Read the model definition and answer for the solid it produces. Units are mm, in the model's axes. A direction names the side the tool comes from. Give positions to 0.01 mm unless a question says otherwise; leave off trailing zeros. Loops run counter-clockwise (first coordinate to the right, second up) from the corner with the lowest first, then second, coordinate; pieces in that order, holes last. Notation, with made-up numbers: (-20.5, 8) - (26.5, 8) arc R17 cw to (26.5, 14) - close; hole circle Ø5 at (34, 47.5). An arc over 180 degrees is marked (long way). Write each question's results on one line, items separated by ' | '. Start each with the question number.
Q1. The part is cut by section A-A, the plane z = 121. Write down the section's boundary in (x, y) (3 decimals), plus the area to 3 significant figures.
Q2. Determine the mould class of faces 3 (the flat face through (1, 6, -127.5)), 4 (the flat face through (-67.875, 6, -2)), 5 (the flat face through (7, 9, -35.25)) for opening direction Z: +Z half, -Z half, draft (parallel to the pull), parting line (faces both ways), or undercut.
Q3. Given pin 1 (3 mm diameter, centred on x = -61, z = -121.5, fed in from +Y); pin 2 (3 mm diameter, centred on x = 33.5, z = -30, fed in from +Y); pin 3 (8 mm diameter, centred on x = -45, z = 54.175, fed in from +Y); pin 4 (5 mm diameter, centred on x = 45.5, z = 55, fed in from +Y), each flat-ended and moving along its own axis, determine where each tip first touches the part or whether it passes through.
Q4. Find the intervals of material crossed by line 1 (X direction, y = 4.55, z = 30) (3 decimals); line 2 (X direction, y = 7.5, z = 121) (3 decimals); line 3 (Z direction, x = 19, y = 5.25), in increasing order. Write a range as from..to.
Q5. For faces 1 (the flat face through (-45, 5.5, -54)), 2 (the flat face through (-31, 11.5, -2)), determine the directions among +Z, -Z, +X, -X, +Y, -Y from which every point of the face is accessible in a straight line to the end or side of a thin tool.
Q6. The part is cut by section C-C, the plane x = 1.5. Write down the section's boundary in (y, z).
Q7. The part is cut by section B-B, the plane x = -45. Write down the section's boundary in (y, z).
```python
from build123d import *

# Parameters (mm, degrees)
BOSS_EXTRUDE1_DEPTH     = 11.5
SKETCH4_R               = 3.075
CUT_EXTRUDE1_DEPTH      = 6
CUT_EXTRUDE6_DEPTH      = 4.6
CUT_EXTRUDE3_DEPTH      = 145.605932192
CUT_EXTRUDE3_DEPTH_BACK = 3.7
SKETCH24_W              = 82.375
SKETCH24_H              = 54
SKETCH25_R              = 1.35
CUT_EXTRUDE4_DEPTH      = 5
CHAMFER4_SIZE           = 0.5
FILLET1_R               = 2
BOSS_EXTRUDE2_DEPTH     = 0.8
CHAMFER5_SIZE           = 0.75


with BuildPart() as part:
    # Sketch1 → Boss-Extrude1 (new body)
    with BuildSketch(Plane(origin=(0, 0, 0), x_dir=(1, 0, 0), z_dir=(0, 1, 0))):
        with BuildLine():
            Line((-67.875, 112.5), (-67.875, -112.5))
            Line((-67.875, -112.5), (-67.875, -125.5))
            ThreePointArc((-67.875, -125.5), (-67.289213562, -126.914213562), (-65.875, -127.5))
            Line((-65.875, -127.5), (65.875, -127.5))
            ThreePointArc((65.875, -127.5), (67.289213562, -126.914213562), (67.875, -125.5))
            Line((67.875, -125.5), (67.875, -112.5))
            Line((67.875, -112.5), (67.875, 112.5))
            Line((67.875, 112.5), (67.875, 125.5))
            ThreePointArc((67.875, 125.5), (67.289213562, 126.914213562), (65.875, 127.5))
            Line((65.875, 127.5), (-65.875, 127.5))
            ThreePointArc((-65.875, 127.5), (-67.289213562, 126.914213562), (-67.875, 125.5))
            Line((-67.875, 125.5), (-67.875, 112.5))
        make_face()
    extrude(amount=BOSS_EXTRUDE1_DEPTH)

    # Sketch4 → Cut-Extrude1 (cut)
    with BuildSketch(Plane(origin=(0, 11.5, 0), x_dir=(1, 0, 0), z_dir=(0, 1, 0))):
        with Locations(Location((-59.875, -121, 0), (0, 0, 270))):
            Circle(SKETCH4_R)
        with Locations(Location((59.875, -121, 0), (0, 0, 270))):
            Circle(SKETCH4_R)
        with Locations(Location((59.875, 121, 0), (0, 0, 270))):
            Circle(SKETCH4_R)
        with Locations(Location((-59.875, 121, 0), (0, 0, 270))):
            Circle(SKETCH4_R)
        with Locations(Location((45, -54.175, 0), (0, 0, 270))):
            Circle(SKETCH4_R)
        with Locations(Location((-45, -54.175, 0), (0, 0, 270))):
            Circle(SKETCH4_R)
        with Locations(Location((45, 54.175, 0), (0, 0, 270))):
            Circle(SKETCH4_R)
        with Locations(Location((-45, 54.175, 0), (0, 0, 270))):
            Circle(SKETCH4_R)
    extrude(amount=-CUT_EXTRUDE1_DEPTH, mode=Mode.SUBTRACT)

    # Sketch21 → Cut-Extrude6 (cut)
    with BuildSketch(Plane(origin=(0, 11.5, 0), x_dir=(1, 0, 0), z_dir=(0, 1, 0))):
        Polygon((67.875, 31), (67.875, -31), (67.875, -31.25), (42.603553391, -31.25), (38.603553391, -35.25), (-22.75, -35.25), (-22.75, 35.25), (38.603553391, 35.25), (42.603553391, 31.25), (67.875, 31.25), align=None)
    extrude(amount=-CUT_EXTRUDE6_DEPTH, mode=Mode.SUBTRACT)

    # Sketch24 → Cut-Extrude3 (cut, two sides: drawn at the far end of the back side and taken through both)
    with BuildSketch(Plane(origin=(0, 6.9, 0), x_dir=(1, 0, 0), z_dir=(0, 1, 0)).offset(-CUT_EXTRUDE3_DEPTH_BACK)):
        with Locations((26.6875, 0)):
            Rectangle(SKETCH24_W, SKETCH24_H)
    extrude(amount=CUT_EXTRUDE3_DEPTH + CUT_EXTRUDE3_DEPTH_BACK, mode=Mode.SUBTRACT)

    # Sketch25 → Cut-Extrude4 (cut)
    with BuildSketch(Plane(origin=(0, 6.9, 0), x_dir=(1, 0, 0), z_dir=(0, 1, 0))):
        with Locations(Location((33.5, 30, 0), (0, 0, 270))):
            Circle(SKETCH25_R)
        with Locations(Location((-17.5, 30, 0), (0, 0, 270))):
            Circle(SKETCH25_R)
        with Locations(Location((33.5, -30, 0), (0, 0, 270))):
            Circle(SKETCH25_R)
        with Locations(Location((-17.5, -30, 0), (0, 0, 270))):
            Circle(SKETCH25_R)
    extrude(amount=-CUT_EXTRUDE4_DEPTH, mode=Mode.SUBTRACT)

    # Chamfer4
    chamfer4_edges = [part.edges().sort_by_distance(p)[0] for p in [
        (-17.5, 6.9, -31.35),
        (33.5, 6.9, 28.65),
        (-17.5, 6.9, 28.65),
        (33.5, 6.9, -31.35),
    ]]
    chamfer(chamfer4_edges, length=CHAMFER4_SIZE)

    # Fillet1
    fillet1_edges = [part.edges().sort_by_distance(p)[0] for p in [
        (26.6875, 3.2, -27),
        (-14.5, 5.05, -27),
        (-14.5, 3.2, 0),
        (-14.5, 5.05, 27),
        (26.6875, 3.2, 27),
    ]]
    fillet(fillet1_edges, radius=FILLET1_R)

    # Sketch26 → Boss-Extrude2 (add)
    with BuildSketch(Plane(origin=(0, 6.9, 0), x_dir=(1, 0, 0), z_dir=(0, 1, 0))):
        Polygon((38.603553391, 35.25), (38.603553391, 27), (67.875, 27), (67.875, 31.25), (42.603553391, 31.25), align=None)
        Polygon((42.603553391, -31.25), (38.603553391, -35.25), (38.603553391, -27), (67.875, -27), (67.875, -31.25), align=None)
    extrude(amount=BOSS_EXTRUDE2_DEPTH)

    # Chamfer5
    chamfer5_edges = [part.edges().sort_by_distance(p)[0] for p in [
        (59.875, 11.5, 117.925),
        (59.875, 11.5, -124.075),
        (45, 11.5, 51.1),
        (-45, 11.5, 51.1),
        (-45, 11.5, -57.25),
        (45, 11.5, -57.25),
        (-59.875, 11.5, -124.075),
        (-59.875, 11.5, 117.925),
    ]]
    chamfer(chamfer5_edges, length=CHAMFER5_SIZE)


solid = part.part
```
Check sheet entries:
1) outline: (-67.875, 0) - (67.875, 0) - (67.875, 11.5) - (63.7, 11.5) - (62.95, 10.75) - (62.95, 5.5) - (56.8, 5.5) - (56.8, 10.75) - (56.05, 11.5) - (-56.05, 11.5) - (-56.8, 10.75) - (-56.8, 5.5) - (-62.95, 5.5) - (-62.95, 10.75) - (-63.7, 11.5) - (-67.875, 11.5) - close | area: 1,490 mm^2
2) face 3: -Z half | face 4: draft | face 5: undercut
3) pin 1: stops at y = 5.5 | pin 2: stops at y = 6.55 | pin 3: stops at y = 11.5 | pin 4: stops at y = 11.14
4) line 1: x = -67.875..-18.85, -16.15..32.15, 34.85..67.875 | line 2: x = -67.875..-62.95, -56.8..56.8, 62.95..67.875 | line 3: z = -127.5..-27, 27..127.5
5) face 1: +Y | face 2: +Z, -Z, +X, -X, +Y
6) outline: (0, -127.5) - (11.5, -127.5) - (11.5, -35.25) - (6.9, -35.25) - (6.9, -27) - (5.2, -27) arc R2 cw to (3.2, -25) - (3.2, 25) arc R2 cw to (5.2, 27) - (6.9, 27) - (6.9, 35.25) - (11.5, 35.25) - (11.5, 127.5) - (0, 127.5) - close
7) outline: (0, -127.5) - (11.5, -127.5) - (11.5, -58) - (10.75, -57.25) - (5.5, -57.25) - (5.5, -51.1) - (10.75, -51.1) - (11.5, -50.35) - (11.5, 50.35) - (10.75, 51.1) - (5.5, 51.1) - (5.5, 57.25) - (10.75, 57.25) - (11.5, 58) - (11.5, 127.5) - (0, 127.5) - close
